Here's how the part is built. I have some questions about the finished solid (model axes, mm). A direction names the side the tool comes from. Round coordinates to 2 decimals unless told otherwise and drop trailing zeros. Write each loop counter-clockwise with the first axis right and the second up, starting at its lowest first coordinate (ties: lowest second). Pieces come first, ordered by that corner, then holes. Notation, with made-up numbers: (80, 1.5) -> (103, 1.5) arc R22 cw to (103, 19.5) -> close; hole circle Ø8 at (67.25, 84.5). An arc over 180 degrees is marked (long way). Answer as CSV lines item,"result".
from build123d import *

# Parameters (mm, degrees)
SKIZZE1_R                       = 1.25
SKIZZE1_R_2                     = 5
AUFSATZ_LINEAR_AUSTRAGEN1_DEPTH = 0.825
VERRUNDUNG1_R                   = 1.5
SKIZZE3_R                       = 5
SKIZZE3_R_2                     = 4
AUFSATZ_LINEAR_AUSTRAGEN2_DEPTH = 1.65
SKIZZE4_R                       = 2.5
SCHNITT_LINEAR_AUSTRAGEN1_DEPTH = 2.65


with BuildPart() as part:
    # Skizze1 → Aufsatz-Linear austragen1 (new body, symmetric)
    with BuildSketch(Plane(origin=(0, 0, 0), x_dir=(1, 0, 0), z_dir=(0, 1, 0))):
        Polygon((-6, 11.6), (-6, 13.3), (6, 13.3), (6, 11.6), (15, 11.6), (15, -11.6), (6, -11.6), (6, -13.3), (-6, -13.3), (-6, -11.6), (-15, -11.6), (-15, 11.6), align=None)
        with Locations((0, -8)):
            Circle(SKIZZE1_R, mode=Mode.SUBTRACT)
        with Locations((0, 8)):
            Circle(SKIZZE1_R, mode=Mode.SUBTRACT)
        Circle(SKIZZE1_R_2, mode=Mode.SUBTRACT)
    extrude(amount=AUFSATZ_LINEAR_AUSTRAGEN1_DEPTH, both=True)

    # Verrundung1
    verrundung1_edges = [part.edges().sort_by_distance(p)[0] for p in [
        (-6, 0, 11.6),
        (-6, 0, -11.6),
        (6, 0, -11.6),
        (6, 0, 11.6),
    ]]
    fillet(verrundung1_edges, radius=VERRUNDUNG1_R)

    # Skizze3 → Aufsatz-Linear austragen2 (add)
    with BuildSketch(Plane(origin=(0, 0.825, 0), x_dir=(1, 0, 0), z_dir=(0, 1, 0))):
        Circle(SKIZZE3_R)
        Circle(SKIZZE3_R_2, mode=Mode.SUBTRACT)
    extrude(amount=-AUFSATZ_LINEAR_AUSTRAGEN2_DEPTH)

    # Skizze4 → Schnitt-Linear austragen1 (cut, through all)
    with BuildSketch(Plane(origin=(0, 0.825, 0), x_dir=(1, 0, 0), z_dir=(0, 1, 0))):
        with Locations((0, 8)):
            Circle(SKIZZE4_R)
        with Locations((0, -8)):
            Circle(SKIZZE4_R)
    extrude(amount=-SCHNITT_LINEAR_AUSTRAGEN1_DEPTH, mode=Mode.SUBTRACT)


solid = part.part
Item 1: Will these pins go through, and if not, where does the flat tip stop? pin 1 (0.5 mm diameter, centred on x = -11.5, y = 0.5, fed in from +Z); pin 2 (5 mm diameter, centred on x = 0, z = 0, fed in from +Y); pin 3 (12 mm diameter, centred on x = -2.5, z = 2, fed in from -Y) (3 decimals); pin 4 (0.5 mm diameter, centred on x = 11.5, y = 0.5, fed in from -Z).
Results found:
pin 1,"stops at z = 11.6"
pin 2,"passes through"
pin 3,"stops at y = -0.825"
pin 4,"stops at z = -11.6"
Item 2: Suppose I cut it at D-D, the plane z = 0. List the corners of the cut face in (x, y) for me (3 decimals).
Results found:
outline,"(-15, -0.825) -> (-4, -0.825) -> (-4, 0.825) -> (-15, 0.825) -> close; (4, -0.825) -> (15, -0.825) -> (15, 0.825) -> (4, 0.825) -> close"
Item 3: Suppose I cut it at C-C, the plane y = 0.25. List the corners of the cut face in (x, z) for me.
Results found:
outline,"(-15, -11.6) -> (-7.5, -11.6) arc R1.5 cw to (-6, -13.1) -> (-6, -13.3) -> (6, -13.3) -> (6, -13.1) arc R1.5 cw to (7.5, -11.6) -> (15, -11.6) -> (15, 11.6) -> (7.5, 11.6) arc R1.5 cw to (6, 13.1) -> (6, 13.3) -> (-6, 13.3) -> (-6, 13.1) arc R1.5 cw to (-7.5, 11.6) -> (-15, 11.6) -> close; hole circle Ø8 at (0, 0); hole circle Ø5 at (0, -8); hole circle Ø5 at (0, 8)"
Item 4: Suppose I cut it at A-A, the plane x = 0. List the corners of the cut face in (y, z) for me (3 decimals), then the cut area to 3 significant figures.
Results found:
outline,"(-0.825, -13.3) -> (0.825, -13.3) -> (0.825, -10.5) -> (-0.825, -10.5) -> close; (-0.825, -5.5) -> (0.825, -5.5) -> (0.825, -4) -> (-0.825, -4) -> close; (-0.825, 4) -> (0.825, 4) -> (0.825, 5.5) -> (-0.825, 5.5) -> close; (-0.825, 10.5) -> (0.825, 10.5) -> (0.825, 13.3) -> (-0.825, 13.3) -> close"
area,"14.2 mm²"
Item 5: Suppose I cut it at B-B, the plane z = -8. List the corners of the cut face in (x, y) for me (3 decimals), then the cut area to 4 significant figures.
Results found:
outline,"(-15, -0.825) -> (-2.5, -0.825) -> (-2.5, 0.825) -> (-15, 0.825) -> close; (2.5, -0.825) -> (15, -0.825) -> (15, 0.825) -> (2.5, 0.825) -> close"
area,"41.25 mm²"
Item 6: I need wall thicknesses on L1, parallel to Z at x = 0, y = -0.2; L2, parallel to X at y = 0.4, z = 8; L3, parallel to X at y = 0.2, z = 0. Which ranges of each line are inside material? Lowest first, please.
Results found:
L1,"z = -13.3 to -10.5, -5.5 to -4, 4 to 5.5, 10.5 to 13.3"
L2,"x = -15 to -2.5, 2.5 to 15"
L3,"x = -15 to -4, 4 to 15"
Item 7: For faces 1 (the flat face through (11, 0, 11.6)), 2 (the flat face through (-11, 0, -11.6)), 3 (the cylindrical face through (-0.54, 0.01, 10.44)), 4 (the flat face through (11, 0, -11.6)), which set-ups out of +Z, -Z, +X, -X, +Y, -Y let a thin tool reach every point of the face, with its end or its side?
Results found:
face 1,"+Z, +X, +Y, -Y"
face 2,"-Z, -X, +Y, -Y"
face 3,"+Y, -Y"
face 4,"-Z, +X, +Y, -Y"
Item 8: If we mould it in two halves opening along Z, with no side actions, what happens to faces 5 (the flat face through (-11, 0, 11.6)), 6 (the cylindrical face through (-0.54, 0.01, -5.56)), 7 (the flat face through (0, 0, -13.3))? For each: pulls with the +Z half, pulls with the -Z half, needs draft (parallel to the pull), parting line crosses it, or undercut.
Results found:
face 5,"pulls with the +Z half"
face 6,"undercut"
face 7,"pulls with the -Z half"
